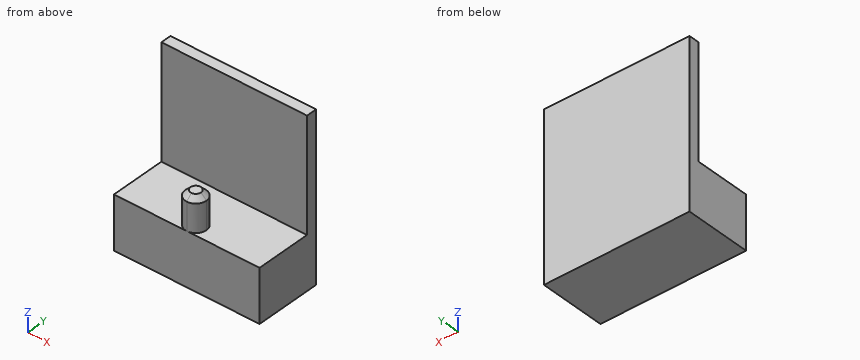
```python
from build123d import *

# Parameters (mm, degrees)
F0_W     = 22
F0_H     = 1.6
F1_DEPTH = 8
F2_DEPTH = 25
F3_DEPTH = 13
F4_SIZE  = 0.8


with BuildPart() as f1:
    # F0 (on Top) → F1 (new body)
    with BuildSketch(Plane.XY):
        Polygon((-15.6633, 3.458741), (-4.6633, 3.458741), (-4.6633, 11.858741), (-26.6633, 11.858741), (-26.6633, 3.458741), align=None)
        with BuildLine():
            ThreePointArc((-14.0633, 5.058741), (-14.531929, 3.92737), (-15.6633, 3.458741))
            ThreePointArc((-15.6633, 3.458741), (-16.794671, 6.190112), (-14.0633, 5.058741))
        make_face(mode=Mode.SUBTRACT)
        with Locations((-15.6633, 12.658741)):
            Rectangle(F0_W, F0_H)
        with BuildLine():
            ThreePointArc((-14.0633, 5.058741), (-16.794671, 6.190112), (-15.6633, 3.458741))
            ThreePointArc((-15.6633, 3.458741), (-14.531929, 3.92737), (-14.0633, 5.058741))
        make_face()
    extrude(amount=F1_DEPTH)

    # F0 (on Top) → F2 (join)
    with BuildSketch(Plane.XY):
        with Locations((-15.6633, 12.658741)):
            Rectangle(F0_W, F0_H)
    extrude(amount=F2_DEPTH)

    # F0 (on Top) → F3 (join)
    with BuildSketch(Plane.XY):
        with BuildLine():
            ThreePointArc((-14.0633, 5.058741), (-16.794671, 6.190112), (-15.6633, 3.458741))
            ThreePointArc((-15.6633, 3.458741), (-14.531929, 3.92737), (-14.0633, 5.058741))
        make_face()
    extrude(amount=F3_DEPTH)

    # F4
    f4_edges = [f1.edges().sort_by_distance(p)[0] for p in [
        (-15.6633, 6.658741, 13),
    ]]
    chamfer(f4_edges, length=F4_SIZE)


solid = f1.part
```
Could you check a few things on this model? Use its own coordinates, in mm. Give positions to 0.01 mm unless a question says otherwise; leave off trailing zeros. Write each loop counter-clockwise with the first axis right and the second up, starting at its lowest first coordinate (ties: lowest second). Pieces come first, ordered by that corner, then holes. Notation, with made-up numbers: (-28, 28.25) - (24, 28.25) arc R23 cw to (24, 50.25) - close; hole circle Ø4 at (0, -22.5). An arc over 180 degrees is marked (long way). One line per item, written item: value. Start each with the question number.
Item 1: Please list where these lines run through material, in increasing order: line 1 (Z direction, x = -10.5, y = 8.5); line 2 (Y direction, x = -9, z = 13.25); line 3 (Y direction, x = -16.25, z = 12.5). Write a range as from..to.
Item 2: Imagine slicing it at A-A, the plane x = -23. List the corners of the cut face in (y, z) for me, and give its area (3 significant figures).
Item 3: Imagine slicing it at C-C, the plane y = 7.75. List the corners of the cut face in (x, z) for me.
Item 4: Imagine slicing it at B-B, the plane z = 23. List the corners of the cut face in (x, y) for me.
Item 5: I'm going to push flat-ended pins straight in: pin 1 (2 mm diameter, centred on x = -18, z = 22, fed in from -Y); pin 2 (3 mm diameter, centred on y = 10.5, z = 18, fed in from +X); pin 3 (0.8 mm diameter, centred on x = -15.5, y = 4.5, fed in from +Z). Where does each tip first touch, or does it pass through?
Geometry says:
1. line 1: 0..8
1. line 2: 11.86..13.46
1. line 3: 3.9..6.22, 11.86..13.46
2. outline: (3.46, 0) - (13.46, 0) - (13.46, 25) - (11.86, 25) - (11.86, 8) - (3.46, 8) - close
2. area: 107 mm^2
3. outline: (-26.66, 0) - (-4.66, 0) - (-4.66, 8) - (-26.66, 8) - close
4. outline: (-26.66, 11.86) - (-4.66, 11.86) - (-4.66, 13.46) - (-26.66, 13.46) - close
5. pin 1: y = 11.86
5. pin 2: x = -4.66
5. pin 3: z = 13
